Solid Edge part; units mm, degrees
sketch "Sketch1" plane through (0, 0, 0) normal (0, 0, 1) x (1, 0, 0)
  arc A0 (-282.5, -10) -> (-282.5, 10) centre (-282.5, 0) cw
  line L0 (-282.5, 10) -> (282.5, 10)
  arc A1 (282.5, 10) -> (282.5, -10) centre (282.5, 0) cw
  line L1 (282.5, -10) -> (-282.5, -10)
  circle A2 centre (-282.5, 0) radius 5
  circle A3 centre (282.5, 0) radius 5
  circle A4 centre (0, 0) radius 5
  dimension "D1" = 282.5
  dimension "D2" = 282.5
extrude "Protrusion1" add sketch "Sketch1" against normal blind 5
fillet "Round_1" radius 1 8 edges at (0, 10, -5) (0, 10, 0) (0, -10, 0) (0, -10, -5) (-292.5, 0, 0) (-292.5, 0, -5) (292.5, 0, 0) (292.5, 0, -5)
properties material "Stainless steel"
Here's how the part is built. I have some questions about the finished solid (model axes, mm). Give positions to 0.01 mm unless a question says otherwise; leave off trailing zeros. Order: outer loops, then holes, each group sorted by start corner. A loop starts at its lowest first (then second) coordinate and runs counter-clockwise, first axis right, second up. Notation, with made-up numbers: (81.5, -24) -> (113.5, -24) arc R29 cw to (113.5, 8) -> close; hole circle Ø2 at (46.25, 19). An arc over 180 degrees is marked (long way). Use CSV: the item, a comma, the result in double quotes. Start each with the question number.
Item 1: Thinking about a two-plate mould opening in Y: for faces 1 (the flat face through (4, 4, 0)), 2 (the cylindrical face through (-292.5, 0.2, -2.5)), 3 (the cylindrical face through (-277.73, 1.5, -2.46)), which applies, pulls with the +Y half, pulls with the -Y half, needs draft (parallel to the pull), parting line crosses it, or undercut?
Item 2: Suppose I cut it at A-A (x = 0). List the corners of the cut face in (y, z) for me.
Item 3: Suppose I cut it at C-C (y = 0). List the corners of the cut face in (x, z) for me.
Item 4: I'm going to push a flat-ended pin straight in: P1, Ø8, axis at x = -282.5, y = 0, coming from the -Z side. Where does the tip first touch, or does it pass through?
Item 5: If I drill on probe 1 along X at (y, z) = (1, -3.8); probe 2 along Y at (x, z) = (-282.5, -1.8); probe 3 along X at (y, z) = (-2.5, -3.85), over which ranges is the centre line in solid material (lowest first)? Write a range as [from, to].
Item 6: Suppose I cut it at B-B (z = -2). List the corners of the cut face in (x, y) for me.
Answer block:
1,face 1,"needs draft"
1,face 2,"parting line crosses it"
1,face 3,"undercut"
2,outline,"(-10, -4) arc R1 ccw to (-9, -5) -> (-5, -5) -> (-5, 0) -> (-9, 0) arc R1 ccw to (-10, -1) -> close; (5, -5) -> (9, -5) arc R1 ccw to (10, -4) -> (10, -1) arc R1 ccw to (9, 0) -> (5, 0) -> close"
3,outline,"(-292.5, -4) arc R1 ccw to (-291.5, -5) -> (-287.5, -5) -> (-287.5, 0) -> (-291.5, 0) arc R1 ccw to (-292.5, -1) -> close; (-277.5, -5) -> (-5, -5) -> (-5, 0) -> (-277.5, 0) -> close; (5, -5) -> (277.5, -5) -> (277.5, 0) -> (5, 0) -> close; (287.5, -5) -> (291.5, -5) arc R1 ccw to (292.5, -4) -> (292.5, -1) arc R1 ccw to (291.5, 0) -> (287.5, 0) -> close"
4,P1,"passes through"
5,probe 1,"x = [-292.45, -287.4], [-277.6, -4.9], [4.9, 277.6], [287.4, 292.45]"
5,probe 2,"y = [-10, -5], [5, 10]"
5,probe 3,"x = [-292.18, -286.83], [-278.17, -4.33], [4.33, 278.17], [286.83, 292.18]"
6,outline,"(-282.5, -10) -> (282.5, -10) arc R10 ccw to (282.5, 10) -> (-282.5, 10) arc R10 ccw to start; hole circle Ø10 at (-282.5, 0); hole circle Ø10 at (0, 0); hole circle Ø10 at (282.5, 0)"
